from build123d import *

# Parameters (mm, degrees)
ESQUISSE2_W             = 91
ESQUISSE2_H             = 6
BOSS_EXTRU_1_DEPTH      = 6
BOSS_EXTRU_1_2_DEPTH    = 6
BOSS_EXTRU_2_DEPTH      = 22
ESQUISSE4_W             = 20
ESQUISSE4_H             = 6
ENL_V_MAT_EXTRU_1_DEPTH = 6
ESQUISSE5_W             = 6
ESQUISSE5_H             = 16
ENL_V_MAT_EXTRU_2_DEPTH = 6


with BuildPart() as part:
    # Esquisse2 → Boss.-Extru.1 (new body)
    with BuildSketch(Plane(origin=(0, 22.295844579, 0), x_dir=(1, 0, 0), z_dir=(0, 1, 0))):
        with Locations((-57.503078089, -203.00005)):
            Rectangle(ESQUISSE2_W, ESQUISSE2_H)
    extrude(amount=BOSS_EXTRU_1_DEPTH)



with BuildPart() as body_2:
    # Esquisse2 → Boss.-Extru.1 2 (new body)
    with BuildSketch(Plane(origin=(0, 22.295844579, 0), x_dir=(1, 0, 0), z_dir=(0, 1, 0))):
        with Locations((53.496921911, -203.00005)):
            Rectangle(ESQUISSE2_W, ESQUISSE2_H)
    extrude(amount=BOSS_EXTRU_1_2_DEPTH)


with BuildPart() as part_1:
    add(part.part)

    add(body_2.part)  # Boss.-Extru.2 merges body 2
    # Esquisse3 → Boss.-Extru.2 (add)
    with BuildSketch(Plane(origin=(0, 0, 200.00005), x_dir=(-1, 0, 0), z_dir=(0, 0, -1))):
        Polygon((-7.996921911, 28.295844579), (12.003078089, 28.295844579), (103.003078089, 28.295844579), (103.003078089, 22.295844579), (12.003078089, 22.295844579), (-7.996921911, 22.295844579), (-98.996921911, 22.295844579), (-98.996921911, 28.295844579), align=None)
    extrude(amount=BOSS_EXTRU_2_DEPTH)

    # Esquisse4 → Enlèv. mat.-Extru.1 (cut)
    with BuildSketch(Plane(origin=(0, 28.295844579, 0), x_dir=(1, 0, 0), z_dir=(0, 1, 0))):
        with Locations((-2.003078089, -203.00005)):
            Rectangle(ESQUISSE4_W, ESQUISSE4_H)
        with Locations((-2.003078089, -181.00005)):
            Rectangle(ESQUISSE4_W, ESQUISSE4_H)
    extrude(amount=-ENL_V_MAT_EXTRU_1_DEPTH, mode=Mode.SUBTRACT)

    # Esquisse5 → Enlèv. mat.-Extru.2 (cut)
    with BuildSketch(Plane(origin=(0, 28.295844579, 0), x_dir=(1, 0, 0), z_dir=(0, 1, 0))):
        with Locations((95.996921911, -192.00005)):
            Rectangle(ESQUISSE5_W, ESQUISSE5_H)
        with Locations((-100.003078089, -192.00005)):
            Rectangle(ESQUISSE5_W, ESQUISSE5_H)
    extrude(amount=-ENL_V_MAT_EXTRU_2_DEPTH, mode=Mode.SUBTRACT)


solid = part_1.part
Check sheet for the modelled part. Datum: model origin and axes. Units: mm. A direction names the side the tool comes from. Round coordinates to 2 decimals unless told otherwise and drop trailing zeros. Loops run counter-clockwise (first coordinate to the right, second up) from the corner with the lowest first, then second, coordinate; pieces in that order, holes last. Notation, with made-up numbers: M 69,24.25 L 102,24.25 A15 cw 102,46.25 Z; hole C 45.5,-3 d7. An arc over 180 degrees is marked long. One line per item, written item: value.
(1) Sectioned sample at D-D, the plane z = 187.5. Record the cut outline in (x, y), then the cut area to 3 significant figures.
Computed values:
outline: M -97,22.3 L 93,22.3 L 93,28.3 L -97,28.3 Z
area: 1,140 mm^2
(2) Sectioned sample at C-C, the plane x = -5. Record the cut outline in (y, z), then the cut area to 3 significant figures.
Computed values:
outline: M 22.3,184 L 28.3,184 L 28.3,200 L 22.3,200 Z
area: 96.0 mm^2
(3) Sectioned sample at A-A, the plane z = 203. Record the cut outline in (x, y).
Computed values:
outline: M -103,22.3 L -12,22.3 L -12,28.3 L -103,28.3 Z; M 8,22.3 L 99,22.3 L 99,28.3 L 8,28.3 Z
(4) Depth check by flat-ended pin: pin 1 Ø1.5 at (y, z) = (24.5, 195.5) entering from +X. Enter the tip coordinate at first touch or a pass-through.
Computed values:
pin 1: stops at x = 93
(5) Sectioned sample at B-B, the plane y = 25.1. Record the cut outline in (x, z).
Computed values:
outline: M -103,178 L -12,178 L -12,184 L 8,184 L 8,178 L 99,178 L 99,184 L 93,184 L 93,200 L 99,200 L 99,206 L 8,206 L 8,200 L -12,200 L -12,206 L -103,206 L -103,200 L -97,200 L -97,184 L -103,184 Z
(6) Thickness scan on line 1 (X direction, y = 23.45, z = 180.5); line 2 (X direction, y = 22.75, z = 199.5); line 3 (Z direction, x = 4, y = 26.25). Record the ranges inside material, lowest first.
Computed values:
line 1: x = -103 to -12, 8 to 99
line 2: x = -97 to 93
line 3: z = 184 to 200
(7) Release check for a two-part mould opening along Z. For faces 6 (the face through (53, 25, 178)), 7 (the face through (-97.003, 25, 192)), 8 (the face through (-58, 25, 206)) record: +Z half, -Z half, draft (parallel to the pull), parting line (faces both ways), or undercut.
Computed values:
face 6: -Z half
face 7: undercut
face 8: +Z half
(8) Access from +Z, -Z, +X, -X, +Y, -Y to the whole of each face (thin tool, end or side, straight path). Record for faces 1 (the face through (96, 25, 200)), 2 (the face through (-3, 28.296, 192)), 3 (the face through (7.997, 25, 203)), 4 (the face through (-2, 25, 184)), 5 (the face through (-100, 25, 200)).
Computed values:
face 1: +X, +Y, -Y
face 2: +Z, -Z, +X, -X, +Y
face 3: +Z, +Y, -Y
face 4: -Z, +Y, -Y
face 5: -X, +Y, -Y
